```python
from build123d import *

# Parameters (mm, degrees)
SKETCH_R      = 2.45
PAD_DEPTH     = 5
SKETCH001_R   = 4
SKETCH001_R_2 = 2.484206
SKETCH001_R_3 = 2.488042
PAD001_DEPTH  = 9
FILLET_R      = 3
CHAMFER_SIZE  = 1


with BuildPart() as part:
    # Sketch → Pad (new body)
    with BuildSketch(Plane.XY):
        Polygon((189.036612, 104.147994), (157.036612, 97.647994), (157.036612, 81.647994), (189.036612, 75.147994), align=None)
        with Locations((185.036612, 80.147994)):
            Circle(SKETCH_R, mode=Mode.SUBTRACT)
        with Locations((185.036612, 99.147994)):
            Circle(SKETCH_R, mode=Mode.SUBTRACT)
        with BuildLine():
            ThreePointArc((181.036612, 92.147994), (182.536612, 93.647994), (181.036612, 95.147994))
            Line((181.036612, 95.147994), (161.036612, 95.147994))
            ThreePointArc((161.036612, 95.147994), (159.536612, 93.647994), (161.036612, 92.147994))
            Line((181.036612, 92.147994), (161.036612, 92.147994))
        make_face(mode=Mode.SUBTRACT)
        with BuildLine():
            ThreePointArc((181.036612, 84.147994), (182.536612, 85.647994), (181.036612, 87.147994))
            Line((181.036612, 87.147994), (161.036612, 87.147994))
            ThreePointArc((161.036612, 87.147994), (159.536612, 85.647994), (161.036612, 84.147994))
            Line((181.036612, 84.147994), (161.036612, 84.147994))
        make_face(mode=Mode.SUBTRACT)
    extrude(amount=PAD_DEPTH)

    # Sketch001 → Pad001 (join)
    with BuildSketch(Plane.XY.offset(5)):
        with Locations((185.036612, 99.147994)):
            Circle(SKETCH001_R)
        with Locations((185.036612, 99.147994)):
            Circle(SKETCH001_R_2, mode=Mode.SUBTRACT)
        with Locations((185.036612, 80.147994)):
            Circle(SKETCH001_R)
        with Locations((185.036612, 80.147994)):
            Circle(SKETCH001_R_3, mode=Mode.SUBTRACT)
    extrude(amount=-PAD001_DEPTH)

    # Fillet
    fillet_edges = [part.edges().sort_by_distance(p)[0] for p in [
        (189.036612, 104.147994, 2.5),
        (189.036612, 75.147994, 2.5),
        (157.036612, 97.647994, 2.5),
        (157.036612, 81.647994, 2.5),
    ]]
    fillet(fillet_edges, radius=FILLET_R)

    # Chamfer
    chamfer_edges = [part.edges().sort_by_distance(p)[0] for p in [
        (171.036612, 95.147994, 0),
        (171.036612, 92.147994, 0),
        (171.036612, 87.147994, 0),
        (171.036612, 84.147994, 0),
    ]]
    chamfer(chamfer_edges, length=CHAMFER_SIZE)


solid = part.part
```
Check sheet for the modelled part. Datum: model origin and axes. Units: mm. A direction names the side the tool comes from. Round coordinates to 2 decimals unless told otherwise and drop trailing zeros. Loops run counter-clockwise (first coordinate to the right, second up) from the corner with the lowest first, then second, coordinate; pieces in that order, holes last. Notation, with made-up numbers: M 68.25,-18 L 124.25,-18 A34 ccw 124.25,20 Z; hole C 25.5,-36.75 d1. An arc over 180 degrees is marked long. Answer as a JSON object with one key per item and string values.
1. Access from +Z, -Z, +X, -X, +Y, -Y to the whole of each face (thin tool, end or side, straight path). Record for faces 1 (the cylindrical face through (159.537, 93.681, 2.972)), 2 (the flat face through (171.177, 87.655, 0.493)), 3 (the cylindrical face through (157.696, 97.072, 2.535)).
Reply:
{"face 1": "+Z, -Z", "face 2": "-Z", "face 3": "+Z, -Z, -X, +Y"}
2. Section check C-C (z = 0.5). Record the boundary of the cut face in (x, y), plus the area to 3 significant figures.
Reply:
{"outline": "M 157.04,84.1 A3 ccw 159.44,81.16 L 185.44,75.88 A3 ccw 189.04,78.82 L 189.04,100.48 A3 ccw 185.44,103.42 L 159.44,98.14 A3 ccw 157.04,95.2 Z; hole M 161.04,83.65 L 181.04,83.65 A2 ccw 181.04,87.65 L 161.04,87.65 A2 ccw Z; hole M 161.04,91.65 L 181.04,91.65 A2 ccw 181.04,95.65 L 161.04,95.65 A2 ccw Z; hole C 185.04,80.15 d4.9; hole C 185.04,99.15 d4.9", "area": "489 mm²"}
3. Mould release check, pull along X, two halves, no side actions. Record for faces 4 (the cylindrical face through (188.85, 81.35, -1.97)), 5 (the flat face through (157.037, 90, 2)), 6 (the flat face through (171, 92.148, 3)): pulls with the +X half, pulls with the -X half, needs draft (parallel to the pull), parting line crosses it, or undercut.
Reply:
{"face 4": "parting line crosses it", "face 5": "pulls with the -X half", "face 6": "undercut"}
4. Section check D-D (z = -1.75). Record the boundary of the cut face in (x, y).
Reply:
{"outline": "C 185.04,80.15 d8; C 185.04,99.15 d8; hole C 185.04,80.15 d4.98; hole C 185.04,99.15 d4.97"}
5. Section check A-A (x = 165.5). Record the boundary of the cut face in (y, z).
Reply:
{"outline": "M 79.93,0 L 83.15,0 L 84.15,1 L 84.15,5 L 79.93,5 Z; M 87.15,1 L 88.15,0 L 91.15,0 L 92.15,1 L 92.15,5 L 87.15,5 Z; M 95.15,1 L 96.15,0 L 99.37,0 L 99.37,5 L 95.15,5 Z"}
6. Gauge pin test, flat ends, axial feed: P1, Ø2, axis at x = 171, z = 2, coming from the -Y side; P2, Ø3, axis at x = 185.04, y = 99.15, coming from the +Z side; P3, Ø2, axis at y = 81, z = 1.5, coming from the -X side; P4, Ø2, axis at y = 80.5, z = 1, coming from the -X side. Record the tip position at first contact, or that the pin passes through.
Reply:
{"P1": "stops at y = 78.61", "P2": "passes through", "P3": "stops at x = 157.89", "P4": "stops at x = 158.54"}
7. Scan lines: line 1 (Y direction, x = 163, z = 2.75); line 2 (Y direction, x = 163, z = 0.25); line 3 (Y direction, x = 183.5, z = -2). Record each from-to range of solid material in increasing order.
Reply:
{"line 1": "y = 80.44 to 84.15, 87.15 to 92.15, 95.15 to 98.86", "line 2": "y = 80.44 to 83.4, 87.9 to 91.4, 95.9 to 98.86", "line 3": "y = 76.45 to 78.19, 82.1 to 83.84, 95.45 to 97.2, 101.1 to 102.84"}
